Autodesk Inventor part; units mm, degrees
ref_plane "Work Plane2" through (-12.6935, 7.5, -12) normal (0, 1, 0) x (1, 0, 0)
ref_plane "YZ Plane" through (0, 0, 0) normal (1, 0, 0) x (0, 1, 0)
ref_plane "XZ Plane" through (0, 0, 0) normal (0, 1, 0) x (-1, 0, 0)
sketch "Sketch1" plane through (0, 0, 0) normal (0, 0, 1) x (1, 0, 0)
  line L0 (-7.9743, 17.1273) -> (-7.9743, -10.9738)
  line L1 (4.0257, 11.5) -> (4.0257, 9)
  line L2 (4.0257, 9) -> (2.5257, 9)
  line L3 (2.5257, 9) -> (2.5257, -13.5)
  line L4 (2.5257, -13.5) -> (0.5257, -13.5)
  line L5 (0.5257, -13.5) -> (0.5257, -18.5)
  line L6 (4.0257, 11.5) -> (0.5257, 11.5)
  line L7 (0.5257, 11.5) -> (0.5257, 6.5)
  line L8 (0.5257, -2.5) -> (-0.9743, -2.5)
  line L9 (-0.9743, -2.5) -> (-0.9743, -11.3304)
  line L10 (-1.9743, -14.5) -> (-1.9743, -18.5)
  line L11 (-1.9743, -18.5) -> (0.5257, -18.5)
  line L12 (-1.9743, -14.5) -> (-0.9743, -14.5)
  line L13 (-0.9743, -14.5) -> (-0.9743, -11.3304)
  line L14 (0.0257, 6.5) -> (0.0257, 0)
  line L15 (0.5257, 6.5) -> (0.0257, 6.5)
  line L16 (0.0257, 0) -> (0.3257, 0)
  line L17 (0.8257, -0.5) -> (0.8257, -2.5)
  line L18 (0.8257, -2.5) -> (0.5257, -2.5)
  arc A0 (0.8257, -0.5) -> (0.3257, 0) centre (0.3257, -0.5) ccw
  point P0 (0.8257, 0)
  dimension "d6" = 14
  dimension "d7" = 17
  dimension "d8" = 21
  dimension "d10" = 5
  dimension "d11" = 12
  dimension "d12" = 4
  dimension "d13" = 30
  dimension "d14" = 5
  dimension "d18" = 24
  dimension "d19" = 16
  dimension "d20" = 17
  dimension "d21" = 0.8
  dimension "d22" = 2.5
  dimension "d23" = 0.5
revolve "Revolution1" add sketch "Sketch1" angle 360 about axis through (-7.9743, 17.1273, 0) along (0, -1, 0)
sketch "Sketch2" plane through (-7.9743, 11.5, 0) normal (0, 1, 0) x (1, 0, 0)
  circle A0 centre (0, 0) radius 12
  line L0 (6.9282, 12) -> (13.8564, 0)
  line L1 (13.8564, 0) -> (6.9282, -12)
  line L2 (6.9282, -12) -> (-6.9282, -12)
  line L3 (-6.9282, -12) -> (-13.8564, 0)
  line L4 (-13.8564, 0) -> (-6.9282, 12)
  line L5 (-6.9282, 12) -> (6.9282, 12)
  point P0 (7.9743, 0)
  point P1 (0, 12)
extrude "Extrusion1" add sketch "Sketch2" against normal blind 8 contours A0 L0 L1 | A0 L5 L0 | L1 L2 A0 | A0 L4 L5 | L2 L3 A0 | A0 L3 L4
sketch "Sketch3" plane through (0, 0, 0) normal (0, 0, 1) x (1, 0, 0)
  line L0 (2.418, 3.5) -> (5.8821, 3.5)
  line L1 (-1.0461, 11.5) -> (-1.0461, 3.5)
  line L2 (-1.0461, 11.5) -> (5.8821, 11.5)
  line L3 (5.8821, 11.5) -> (5.8821, 3.5)
  line L4 (-21.8307, 3.5) -> (-18.3666, 3.5)
  line L5 (-21.8307, 11.5) -> (-21.8307, 3.5)
  line L6 (-21.8307, 11.5) -> (-14.9025, 11.5)
  line L7 (-14.9025, 11.5) -> (-14.9025, 3.5)
  line L8 (-7.9743, 20.7963) -> (-7.9743, 13.4843)
  line L9 (6.3821, 12) -> (4.1894, 12)
  line L10 (6.3821, 12) -> (6.3821, 10.5)
  line L11 (4.1894, 12) -> (6.3821, 10.5)
  line L12 (-18.3666, 9) -> (-18.3666, 3.5)
  line L13 (-18.3666, 3.5) -> (-14.9025, 3.5)
  line L14 (2.418, 9) -> (2.418, 3.5)
  line L15 (-1.0461, 3.5) -> (2.418, 3.5)
  point P0 (0, 0)
  dimension "d36" = 0.5
  dimension "d38" = 0.5
  dimension "d39" = 1.5
revolve "Revolution2" cut sketch "Sketch3" angle 360 about axis through (-7.9743, 20.7963, 0) along (0, -1, 0) contours L11 L2 L3 | L3 L2 L11 L9 L10
sketch "Sketch5" plane through (0, 0, 0) normal (0, 0, 1) x (1, 0, 0)
  point P0 (0, 0)
ref_plane "Work Plane2" through (-12.6935, 7.5, -12) normal (0, 1, 0) x (1, 0, 0)
mirror "Mirror2" about plane through (-12.6935, 7.5, -12) normal (0, 1, 0) of "Revolution2"
thread "Thread1"
thread "Thread2"
fillet "Fillet1" radius 0.5 1 edges at (-16.4743, -13.5, 0)
fillet "Fillet2" radius 0.5 1 edges at (-18.4743, 9, 0)
properties part number "MUSAB2"
The model under review builds one solid part; all positions refer to its coordinate system, in mm. A direction names the side the tool comes from. Round coordinates to 2 decimals unless told otherwise and drop trailing zeros. Loops run counter-clockwise (first coordinate to the right, second up) from the corner with the lowest first, then second, coordinate; pieces in that order, holes last. Notation, with made-up numbers: M -36.75,24.25 L 3.25,24.25 A33 cw 3.25,59.25 Z; hole C 74.25,69.25 d7. An arc over 180 degrees is marked long. Answer as CSV lines item,"result". Start each with the question number.
Item 1: Consider section B-B (y = -12). Write out the cut boundary in (x, z), then the cut area to 3 significant figures.
Item 2: Mouldability with a two-part tool opening along X and no side actions: class faces 4 (the face through (-1.298, -8.416, -2.103)), 5 (the face through (-2, 3.5, 11)), 6 (the face through (5.194, 3.687, 0.027)), 7 (the face through (-1.9, 6.29, -10.35)) as released by +X, released by -X, zero draft, split by the parting line, or undercut.
Item 3: For faces 1 (the face through (-14, 3.5, 11)), 2 (the face through (-2, 3.5, -11)), 3 (the face through (-3, 9, -10)), list the 3-axis set-ups (+Z, -Z, +X, -X, +Y, -Y) from which the entire face can be reached by the end or side of a thin tool; tool diameter is ignored.
Item 4: Insertion check: P1, Ø8, axis at y = -2.5, z = 5.5, coming from the -X side; P2, Ø1.5, axis at y = -10, z = -5, coming from the +X side; P3, Ø4, axis at y = -6.5, z = -1, coming from the +X side; P4, Ø11, axis at x = -11.5, z = -2.5, coming from the +Y side. Each pin has a flat end and moves straight along its axis. Give the tip position at first contact, or say it passes through.
Item 5: Wall thickness on line 1 (X direction, y = -5, z = -0.25); line 2 (Z direction, x = -16.75, y = 8.5); line 3 (X direction, y = 8.5, z = 7.5): over which ranges is each line inside the solid? List them lowest first. Write a range as [from, to].
Item 6: Consider section C-C (y = 1.5). Write out the cut boundary in (x, z), then the cut area to 3 significant figures.
Answer:
1,outline,"C -7.97,0 d21; hole C -7.97,0 d14"
1,area,"192 mm^2"
2,face 4,"undercut"
2,face 5,"zero draft"
2,face 6,"released by +X"
2,face 7,"undercut"
3,face 1,"+Z, -X, -Y"
3,face 2,"-Z, +X, -Y"
3,face 3,"-Y"
4,P1,"stops at x = -18.37"
4,P2,"stops at x = 1.63"
4,P3,"stops at x = 2.53"
4,P4,"stops at y = 11.5"
5,line 1,"x = [-18.47, -14.97], [-0.98, 2.52]"
5,line 2,"z = [-8.8, -8.18], [-5.77, 5.77], [8.18, 8.8]"
5,line 3,"x = [-17.5, -17.34], [-15.32, -11.97], [-3.97, -0.63], [1.39, 1.55]"
6,outline,"C -7.97,0 d21; hole C -7.97,0 d16"
6,area,"145 mm^2"
